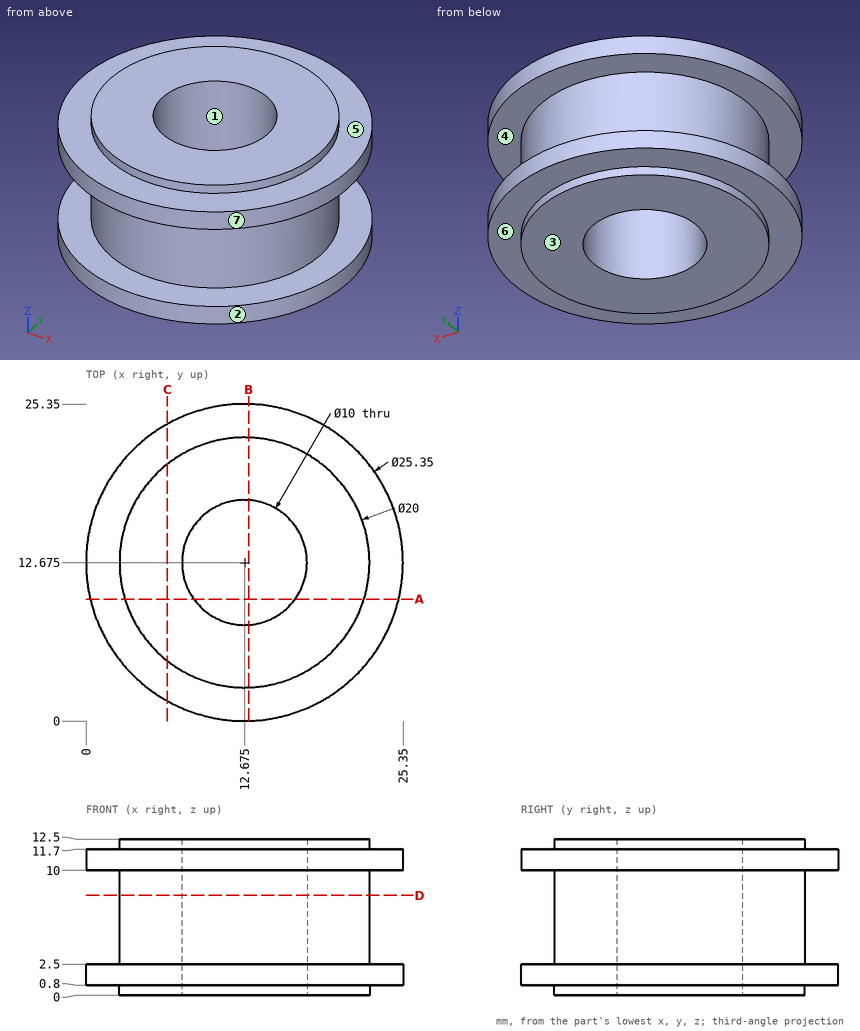
Check sheet for the drawn part. Datum: minimum x, y, z corner. Units: mm. A direction names the side the tool comes from. Give positions to 0.01 mm unless a question says otherwise; leave off trailing zeros. Order: outer loops, then holes, each group sorted by start corner. A loop starts at its lowest first (then second) coordinate and runs counter-clockwise, first axis right, second up. Notation, with made-up numbers: (14.5, -14.75) - (28.5, -14.75) arc R19 ccw to (28.5, 21.25) - close; hole circle Ø6 at (35, 35). An arc over 180 degrees is marked (long way). Write item = value, one per line. Start each with the question number.
1) Section check A-A (y = 9.75). Enter the section's corners in (x, z).
2) Gauge pin test, flat ends, axial feed: pin 1 Ø3 at (x, z) = (21, 11) entering from +Y; pin 2 Ø12.5 at (x, y) = (11, 11.5) entering from -Z; pin 3 Ø5 at (x, z) = (5.5, 5.5) entering from +Y; pin 4 Ø5 at (y, z) = (9, 3.5) entering from -X. Record the tip position at first contact, or that the pin passes through.
3) Section check D-D (z = 8). Enter the section's corners in (x, y) (3 decimals).
4) Scan lines: L1, parallel to Z at x = 10.5, y = 23; L2, parallel to Y at x = 10.75, z = 10.75; L3, parallel to Y at x = 14.5, z = 11.5. Record each from-to range of solid material in increasing order.
5) Draft check along X on the marked faces 1, 2 and 3. Enter one of: released by +X, released by -X, zero draft, split by the parting line, or undercut.
6) Section check B-B (x = 13). Enter the section's corners in (y, z), then the cut area to 3 significant figures.
7) Access from +Z, -Z, +X, -X, +Y, -Y to the whole of each face (thin tool, end or side, straight path). Record for the marked faces 4, 5, 6 and 7.
8) Section check C-C (x = 6.5). Enter the section's corners in (y, z).
Geometry check:
q1.outline = (0.34, 0.8) - (3.11, 0.8) - (3.11, 0) - (8.62, 0) - (8.62, 12.5) - (3.11, 12.5) - (3.11, 11.7) - (0.34, 11.7) - (0.34, 10) - (3.11, 10) - (3.11, 2.5) - (0.34, 2.5) - close; (16.73, 0) - (22.24, 0) - (22.24, 0.8) - (25.01, 0.8) - (25.01, 2.5) - (22.24, 2.5) - (22.24, 10) - (25.01, 10) - (25.01, 11.7) - (22.24, 11.7) - (22.24, 12.5) - (16.73, 12.5) - close
q2.pin_1 = 23.36
q2.pin_2 = 0
q2.pin_3 = 21.51
q2.pin_4 = 0.08
q3.outline = circle Ø20 at (12.675, 12.675); hole circle Ø10 at (12.675, 12.675)
q4.L1 = 0.8 to 2.5, 10 to 11.7
q4.L2 = 0.15 to 8.06, 17.29 to 25.2
q4.L3 = 0.13 to 8.02, 17.33 to 25.22
q5.face_1 = undercut
q5.face_2 = split by the parting line
q5.face_3 = zero draft
q6.outline = (0, 0.8) - (2.68, 0.8) - (2.68, 0) - (7.69, 0) - (7.69, 12.5) - (2.68, 12.5) - (2.68, 11.7) - (0, 11.7) - (0, 10) - (2.68, 10) - (2.68, 2.5) - (0, 2.5) - close; (17.66, 0) - (22.67, 0) - (22.67, 0.8) - (25.35, 0.8) - (25.35, 2.5) - (22.67, 2.5) - (22.67, 10) - (25.35, 10) - (25.35, 11.7) - (22.67, 11.7) - (22.67, 12.5) - (17.66, 12.5) - close
q6.area = 143 mm2
q7.face_4 = none
q7.face_5 = +Z
q7.face_6 = -Z
q7.face_7 = +Z, -Z
q8.outline = (1.61, 0.8) - (4.81, 0.8) - (4.81, 0) - (20.54, 0) - (20.54, 0.8) - (23.74, 0.8) - (23.74, 2.5) - (20.54, 2.5) - (20.54, 10) - (23.74, 10) - (23.74, 11.7) - (20.54, 11.7) - (20.54, 12.5) - (4.81, 12.5) - (4.81, 11.7) - (1.61, 11.7) - (1.61, 10) - (4.81, 10) - (4.81, 2.5) - (1.61, 2.5) - close
